from build123d import *

# Parameters (mm, degrees)
SKETCH_1_R      = 12.5
EXTRUDE_1_DEPTH = 8
CHAMFER_1_SIZE  = 5


with BuildPart() as part:
    # 草图1 → 凸台-拉伸1 (new, symmetric)
    with BuildSketch(Plane(origin=(0, 0, 0), x_dir=(0, 0, -1), z_dir=(1, 0, 0))):
        with BuildLine():
            Line((-22.5, 0), (-22.5, -35))
            Line((-22.5, -35), (-10.783162242, -57.084286562))
            Line((-10.783162242, -57.084286562), (-6.36630493, -54.74091901))
            ThreePointArc((-6.36630493, -54.74091901), (0.393919934, -56.814408771), (-1.679569826, -63.574633635))
            Line((-1.679569826, -63.574633635), (-6.096427139, -65.918001187))
            Line((-6.096427139, -65.918001187), (21.5, -117.932667397))
            ThreePointArc((21.5, -117.932667397), (66.291252117, -94.19847395), (91.981942633, -50.5))
            Line((91.981942633, -50.5), (96.5, -50.5))
            Line((96.5, -50.5), (88.331264802, -13.972315085))
            ThreePointArc((88.331264802, -13.972315085), (86.235037436, -10.344476702), (82.442373664, -8.563723486))
            ThreePointArc((82.442373664, -8.563723486), (46.03018843, 0.843735432), (12.819740934, 18.490652838))
            ThreePointArc((12.819740934, 18.490652838), (-10.435655921, 19.933566803), (-22.5, 0))
        make_face()
        Circle(SKETCH_1_R, mode=Mode.SUBTRACT)
    extrude(amount=EXTRUDE_1_DEPTH, both=True)

    # 倒角1
    chamfer_1_edges = [part.edges().sort_by_distance(p)[0] for p in [
        (-8, -94.19847395, -66.291252117),
        (8, -94.19847395, -66.291252117),
    ]]
    chamfer(chamfer_1_edges, length=CHAMFER_1_SIZE)


solid = part.part
CAD build for the part. Positions are in the model's coordinates, mm. A direction names the side the tool comes from. Round coordinates to 2 decimals unless told otherwise and drop trailing zeros. Loops run counter-clockwise (first coordinate to the right, second up) from the corner with the lowest first, then second, coordinate; pieces in that order, holes last.
(1) Which spindle directions (+Z, -Z, +X, -X, +Y, -Y) get a long thin tool onto all of the face, cutting with end or side? Do faces 5 (the flat face through (0.11, -55.93, 8.61)), 6 (the flat face through (0, -17, 22.5)), 7 (the flat face through (0, -50.5, -94)). Say none if no direction does.
(2) Drop flat-ended pins along their axis: pin 1 (6 mm diameter, centred on x = 4.5, z = -81, fed in from +Y); pin 2 (1 mm diameter, centred on x = 5, y = -76, fed in from -Z); pin 3 (8 mm diameter, centred on x = 1.5, z = -91.5, fed in from -Y). Give the stop position or say it passes through.
(3) Two-plate mould, pull along Y, no slides. Class faces 1 (the flat face through (0.112, -45.888, 16.724)), 2 (the flat face through (8, -44, -36)), 3 (the flat face through (0.11, -64.73, 3.86)), 4 (the cylindrical face through (0.112, 0.653, -46.522)): +Y half, -Y half, draft (parallel to the pull), parting line (faces both ways), or undercut.
(4) Cut at B-B (z = -10). Give the cut face in (x, y).
(5) Wall check: line 1 along Y through (x, z) = (2.25, 0); line 2 along Y through (x, z) = (-5, -4); line 3 along Y through (x, z) = (6.25, -1.5). Give the ranges that are in metal, low to high.
(6) Cut at A-A (y = -3.5). Give the cut face in (x, z), plus the area to 3 significant figures.
Findings below:
1. face 5: +X, -X, -Y
1. face 6: +Z, +X, -X, +Y, -Y
1. face 7: -Z, -Y
2. pin 1: stops at y = -7.9
2. pin 2: stops at z = -79.35
2. pin 3: stops at y = -63.59
3. face 1: -Y half
3. face 2: draft
3. face 3: undercut
3. face 4: +Y half
4. outline: (-8, -96.26) - (8, -96.26) - (8, -7.5) - (-8, -7.5) - close; (-8, 7.5) - (8, 7.5) - (8, 20.16) - (-8, 20.16) - close
5. line 1: y = -77.41 to -62.13, -56.19 to -12.5, 12.5 to 22.5
5. line 2: y = -84.95 to -11.84, 11.84 to 22.14
5. line 3: y = -80.24 to -12.41, 12.41 to 22.45
6. outline: (-8, -58.77) - (8, -58.77) - (8, -12) - (-8, -12) - close; (-8, 12) - (8, 12) - (8, 22.5) - (-8, 22.5) - close
6. area: 916 mm2
